Verification items for the finished model (mm, model axes). Face numbers are marked on the shaded views. A direction names the side the tool comes from. Give positions to 0.01 mm unless a question says otherwise; leave off trailing zeros. Loops run counter-clockwise (first coordinate to the right, second up) from the corner with the lowest first, then second, coordinate; pieces in that order, holes last. Notation, with made-up numbers: (25, 68.25) -> (47, 68.25) arc R11 cw to (47, 77.25) -> close; hole circle Ø3 at (61, 4). An arc over 180 degrees is marked (long way). Answer in a Markdown table with one row per item. Add a question column.
Q1. Section check C-C on z = 2. Enter the section's corners in (x, y).
Q2. Release check for a two-part mould opening along Y. For the marked faces 1, 2, 3 and 4 record: pulls with the +Y half, pulls with the -Y half, needs draft (parallel to the pull), parting line crosses it, or undercut.
Q3. Set-up check for the marked faces 5 and 6: record each of +Z, -Z, +X, -X, +Y, -Y from which the full face is reachable in a straight line by a thin tool's end or side.
Q4. Gauge pin test, flat ends, axial feed: P1, Ø10, axis at y = 51.5, z = 32.5, coming from the -X side; P2, Ø4, axis at x = 22, z = 17, coming from the +Y side; P3, Ø3, axis at y = 57.5, z = 26, coming from the -X side; P4, Ø10, axis at x = 37, y = 46.5, coming from the +Z side. Record the tip position at first contact, or that the pin passes through.
Q5. Section check A-A on x = 0. Enter the section's corners in (y, z), and give its area (3 significant figures).
Q6. Section check B-B on y = 38.1. Enter the section's corners in (x, z), and give its area (4 significant figures).
Q7. Section check D-D on y = 51. Enter the section's corners in (x, z), and give its area (3 significant figures).
Q8. Material ranges on probe 1 along X at (y, z) = (38.1, 13.5); probe 2 along Y at (x, z) = (0, 10); probe 3 along Y at (x, z) = (-28, 24.5), recorded low to high.
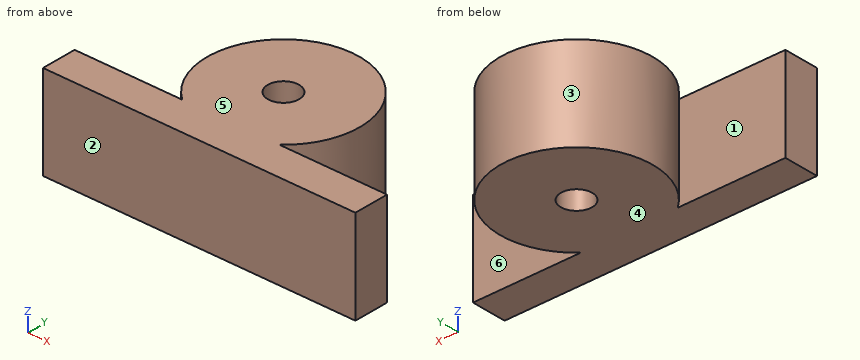
```python
from build123d import *

# Parameters (mm, degrees)
SKETCH1_R           = 30.95625
SKETCH1_R_2         = 6.35
BOSS_EXTRUDE1_DEPTH = 38.1


with BuildPart() as part:
    # Sketch1 → Boss-Extrude1 (new body)
    # profile 1 of 2: a face of its own
    with BuildSketch(Plane.XY):
        with Locations((0, 38.1)):
            Circle(SKETCH1_R)
        with Locations(Location((0, 38.1, 0), (0, 0, 180))):
            Circle(SKETCH1_R_2, mode=Mode.SUBTRACT)
    # profile 2 of 2: a face of its own
    with BuildSketch(Plane.XY):
        with BuildLine():
            Line((-63.5, 14.2875), (-63.5, 0))
            Line((-63.5, 0), (63.5, 0))
            Line((63.5, 0), (63.5, 14.2875))
            Line((63.5, 14.2875), (19.780148074, 14.2875))
            ThreePointArc((19.780148074, 14.2875), (0, 7.14375), (-19.780148074, 14.2875))
            Line((-19.780148074, 14.2875), (-63.5, 14.2875))
        make_face()
    extrude(amount=BOSS_EXTRUDE1_DEPTH)


solid = part.part
```
Taken from the geometry:
| question | item | result |
|---|---|---|
| 1 | outline | (-63.5, 0) -> (63.5, 0) -> (63.5, 14.29) -> (19.78, 14.29) arc R30.96 ccw (long way) to (-19.78, 14.29) -> (-63.5, 14.29) -> close; hole circle Ø12.7 at (0, 38.1) |
| 2 | face 1 | undercut |
| 2 | face 2 | pulls with the -Y half |
| 2 | face 3 | undercut |
| 2 | face 4 | needs draft |
| 3 | face 5 | +Z, +X, -X, +Y, -Y |
| 3 | face 6 | +Z, -Z, +X |
| 4 | P1 | stops at x = -29.79 |
| 4 | P2 | stops at y = 61.73 |
| 4 | P3 | stops at x = -25.26 |
| 4 | P4 | passes through |
| 5 | outline | (0, 0) -> (31.75, 0) -> (31.75, 38.1) -> (0, 38.1) -> close; (44.45, 0) -> (69.06, 0) -> (69.06, 38.1) -> (44.45, 38.1) -> close |
| 5 | area | 2,150 mm² |
| 6 | outline | (-30.96, 0) -> (-6.35, 0) -> (-6.35, 38.1) -> (-30.96, 38.1) -> close; (6.35, 0) -> (30.96, 0) -> (30.96, 38.1) -> (6.35, 38.1) -> close |
| 6 | area | 1,875 mm² |
| 7 | outline | (-28.14, 0) -> (28.14, 0) -> (28.14, 38.1) -> (-28.14, 38.1) -> close |
| 7 | area | 2,140 mm² |
| 8 | probe 1 | x = -30.96 to -6.35, 6.35 to 30.96 |
| 8 | probe 2 | y = 0 to 31.75, 44.45 to 69.06 |
| 8 | probe 3 | y = 0 to 14.29, 24.9 to 51.3 |
